```python
from build123d import *

# Parameters (mm, degrees)
BOSS_EXTRUDE1_DEPTH = 60
SKETCH2_R           = 3
CUT_EXTRUDE1_DEPTH  = 120.268604419


with BuildPart() as part:
    # Sketch1 → Boss-Extrude1 (new body)
    with BuildSketch(Plane.XY):
        Polygon((0, 70), (0, 0), (80, 0), (80, 70), (75, 70), (75, 5), (5, 5), (5, 70), align=None)
    extrude(amount=-BOSS_EXTRUDE1_DEPTH)

    # Sketch2 → Cut-Extrude1 (cut, through all)
    with BuildSketch(Plane(origin=(0, 5, 0), x_dir=(1, 0, 0), z_dir=(0, 1, 0))):
        with Locations(Location((40, 30, 0), (0, 0, 180))):
            Circle(SKETCH2_R)
        with Locations(Location((20, 30, 0), (0, 0, 180))):
            Circle(SKETCH2_R)
        with Locations(Location((40, 45, 0), (0, 0, 180))):
            Circle(SKETCH2_R)
        with Locations((40, 15)):
            Circle(SKETCH2_R)
        with Locations((60, 30)):
            Circle(SKETCH2_R)
    extrude(amount=-CUT_EXTRUDE1_DEPTH, mode=Mode.SUBTRACT)


solid = part.part
```
CAD build for the part. Positions are in the model's coordinates, mm. A direction names the side the tool comes from. Give positions to 0.01 mm unless a question says otherwise; leave off trailing zeros. Write each loop counter-clockwise with the first axis right and the second up, starting at its lowest first coordinate (ties: lowest second). Pieces come first, ordered by that corner, then holes. Notation, with made-up numbers: M 39.25,-12 L 95.25,-12 A19 ccw 95.25,20 Z; hole C -38.5,-28.75 d11. An arc over 180 degrees is marked long. Return JSON: item names as keys, results as strings. Group by question number.
(1) Band-saw the part on A-A (y = 7.5). Give the cut face in (x, z), and give its area (3 significant figures).
(2) Drill centre lines: L1, parallel to Z at x = 40, y = 2; L2, parallel to X at y = 2, z = -15; L3, parallel to X at y = 8.5, z = -42. Where is each one in solid material? Low to high. Write a range as [from, to].
(3) Band-saw the part on C-C (z = -15). Give the cut face in (x, y).
(4) Flat gauge pin, fed straight in: pin 1 Ø7 at (x, z) = (40, -15) entering from +Y. Where does the tip first touch, or does it go through?
(5) Band-saw the part on B-B (x = 40). Give the cut face in (y, z), and give its area (3 significant figures).
(6) 3-axis set-ups, long thin cutter, end or side, ignore diameter. For faces 5 (the face through (43, 3, -30)), 6 (the face through (40, 5, -36)): which of +Z, -Z, +X, -X, +Y, -Y reach the whole face in a straight line?
(7) Band-saw the part on D-D (z = -56). Give the cut face in (x, y).
(8) Mould opens along X. For faces 1 (the face through (37.6, 2.5, -13.2)), 2 (the face through (80, 35, -30)), 3 (the face through (42.21, 2.54, -42.97)), 4 (the face through (78, 70, -30)) say: pulls with the +X half, pulls with the -X half, needs draft (parallel to the pull), parting line crosses it, or undercut.
Entries:
{
 "1": {"outline": "M 0,-60 L 5,-60 L 5,0 L 0,0 Z; M 75,-60 L 80,-60 L 80,0 L 75,0 Z", "area": "600 mm^2"},
 "2": {"L1": "z = [-60, -48], [-42, -33], [-27, -18], [-12, 0]", "L2": "x = [0, 37], [43, 80]", "L3": "x = [0, 5], [75, 80]"},
 "3": {"outline": "M 0,0 L 37,0 L 37,5 L 5,5 L 5,70 L 0,70 Z; M 43,0 L 80,0 L 80,70 L 75,70 L 75,5 L 43,5 Z"},
 "4": {"pin 1": "stops at y = 5"},
 "5": {"outline": "M 0,-60 L 5,-60 L 5,-48 L 0,-48 Z; M 0,-42 L 5,-42 L 5,-33 L 0,-33 Z; M 0,-27 L 5,-27 L 5,-18 L 0,-18 Z; M 0,-12 L 5,-12 L 5,0 L 0,0 Z", "area": "210 mm^2"},
 "6": {"face 5": "+Y, -Y", "face 6": "+Z, -Z, +Y"},
 "7": {"outline": "M 0,0 L 80,0 L 80,70 L 75,70 L 75,5 L 5,5 L 5,70 L 0,70 Z"},
 "8": {"face 1": "undercut", "face 2": "pulls with the +X half", "face 3": "undercut", "face 4": "needs draft"}
}
